Source: three-view drawing plus pictorial views. Frame: mm from the lowest corner of the part. A direction names the side the tool comes from. Coordinates: 2 decimals unless noted, no trailing zeros. Write each loop counter-clockwise with the first axis right and the second up, starting at its lowest first coordinate (ties: lowest second). Pieces come first, ordered by that corner, then holes. Notation, with made-up numbers: (-17.5, 29.25) - (-6.5, 29.25) arc R17 ccw to (-6.5, 51.25) - close; hole circle Ø1 at (89.25, -35). An arc over 180 degrees is marked (long way). Answer as a JSON object with one key per item and string values. Group by question number.
Item 1: Mould query, pull axis Z, two halves, no side actions, for the marked faces 1, 2 and 3. Classes: pulls with the +Z half, pulls with the -Z half, needs draft (parallel to the pull), parting line crosses it, or undercut.
Item 2: Section C-C on y = 17.5. Return loops of the section in (x, z).
Item 3: Section A-A on x = 10. Return loops of the section in (y, z).
Item 4: Section D-D on z = 2. State how many separate pieces and enclosed holes the cut face has, and give its area (3 significant figures).
Item 5: First-contact query: pin 1 Ø1.5 at (x, z) = (10, 1.5) entering from +Y; pin 2 Ø1.2 at (y, z) = (3.5, 2) entering from -X; pin 3 Ø2 at (x, z) = (2.5, 3) entering from -Y. Flat tips, straight axial feed; report the tip coordinate or a pass-through.
Item 6: Line query: line 1 along X through (y, z) = (11.9, 2); line 2 along Y through (x, z) = (3.75, 0.55). Output: solid intervals per line, ascending. Write a range as from..to.
Item 7: Set-up query: the marked faces 4, 5, 6, 7 and 8. Return all of +Z, -Z, +X, -X, +Y, -Y with unobstructed straight access to the full face (end or side cutting, diameter ignored); none if empty.
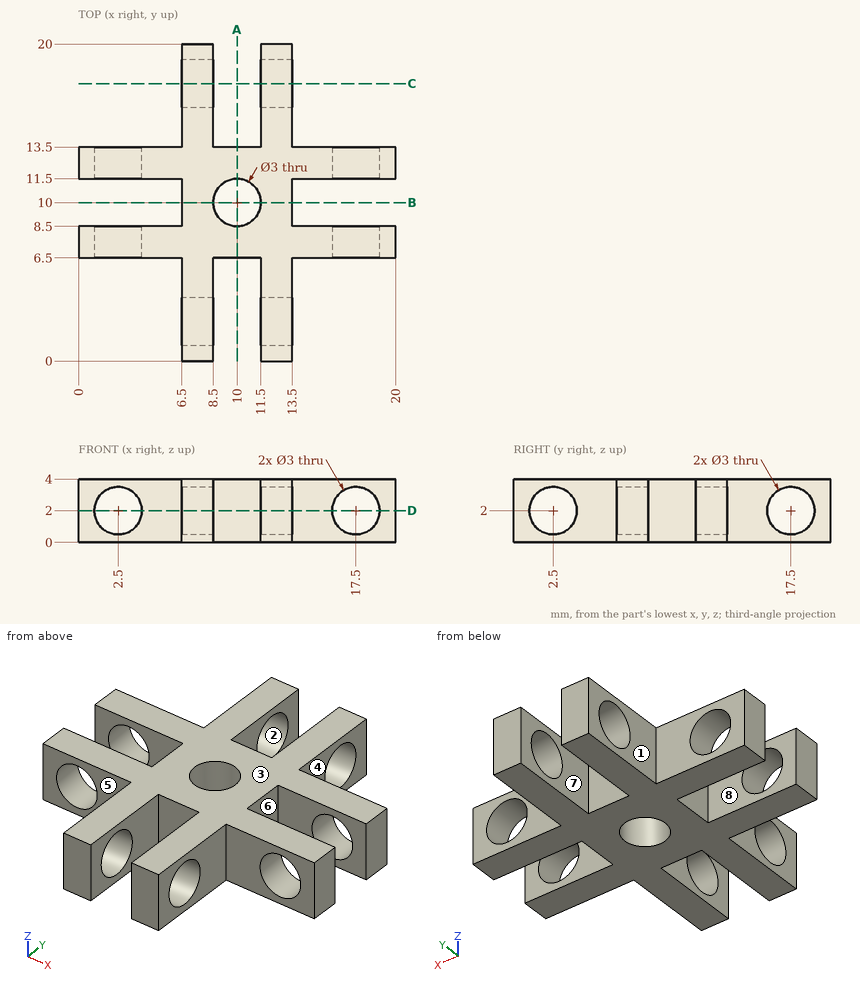
Checks:
{
 "1": {"face 1": "needs draft", "face 2": "undercut", "face 3": "pulls with the +Z half"},
 "2": {"outline": "(6.5, 0) - (8.5, 0) - (8.5, 0.5) - (6.5, 0.5) - close; (6.5, 3.5) - (8.5, 3.5) - (8.5, 4) - (6.5, 4) - close; (11.5, 0) - (13.5, 0) - (13.5, 0.5) - (11.5, 0.5) - close; (11.5, 3.5) - (13.5, 3.5) - (13.5, 4) - (11.5, 4) - close"},
 "3": {"outline": "(6.5, 0) - (8.5, 0) - (8.5, 4) - (6.5, 4) - close; (11.5, 0) - (13.5, 0) - (13.5, 4) - (11.5, 4) - close"},
 "4": {"separate pieces": "9", "enclosed holes": "1", "area": "97.9 mm^2"},
 "5": {"pin 1": "y = 13.5", "pin 2": "x = 6.5", "pin 3": "y = 6.5"},
 "6": {"line 1": "0..1, 4..16, 19..20", "line 2": "6.5..8.5, 11.5..13.5"},
 "7": {"face 4": "+Z, -Z, +X, +Y", "face 5": "+Z, -Z, -X, -Y", "face 6": "+Z, -Z, +X", "face 7": "+Z, -Z, +Y", "face 8": "+Z, -Z, -X"}
}
